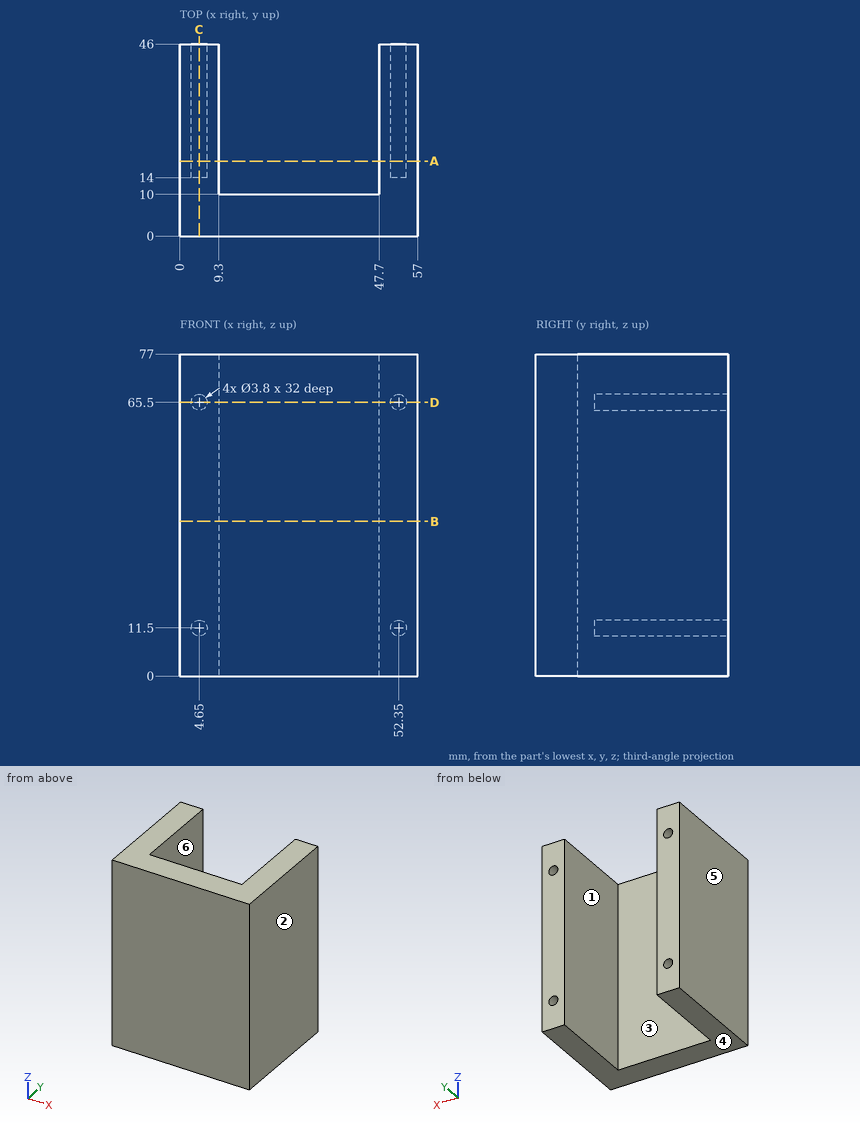
Check sheet for the drawn part. Datum: minimum x, y, z corner. Units: mm. A direction names the side the tool comes from. Give positions to 0.01 mm unless a question says otherwise; leave off trailing zeros. Write each loop counter-clockwise with the first axis right and the second up, starting at its lowest first coordinate (ties: lowest second). Pieces come first, ordered by that corner, then holes.
(1) Access from +Z, -Z, +X, -X, +Y, -Y to the whole of each face (thin tool, end or side, straight path). Record for the marked faces 5 and 6.
(2) Mould release check, pull along X, two halves, no side actions. Record for the marked faces 1, 2, 3 and 4: +X half, -X half, draft (parallel to the pull), parting line (faces both ways), or undercut.
(3) Cross-section at B-B (z = 37). Enter the section's corners in (x, y), plus the area to 3 significant figures.
(4) Cross-section at A-A (y = 18). Enter the section's corners in (x, z), plus the area to 3 significant figures.
(5) Gauge pin test, flat ends, axial feed: pin 1 (4 mm diameter, centred on x = 52, z = 65.5, fed in from +Y); pin 2 (11.5 mm diameter, centred on x = 21.5, z = 49.5, fed in from +Y); pin 3 (2.5 mm diameter, centred on x = 52.35, z = 11.5, fed in from +Y). Record the tip position at first contact, or that the pin passes through.
(6) Cross-section at D-D (z = 65.5). Enter the section's corners in (x, y).
(7) Cross-section at C-C (x = 4.65). Enter the section's corners in (y, z), plus the area to 3 significant figures.
(8) Material ranges on line 1 (X direction, y = 35, z = 65.5); line 2 (X direction, y = 39.5, z = 34.5); line 3 (Z direction, x = 4.5, y = 23.5), recorded low to high.
Worked out:
1. face 5: +Z, -Z, -X, +Y, -Y
1. face 6: +Z, -Z, +Y
2. face 1: undercut
2. face 2: +X half
2. face 3: undercut
2. face 4: draft
3. outline: (0, 0) - (57, 0) - (57, 46) - (47.7, 46) - (47.7, 10) - (9.3, 10) - (9.3, 46) - (0, 46) - close
3. area: 1,240 mm2
4. outline: (0, 0) - (9.3, 0) - (9.3, 77) - (0, 77) - close; (47.7, 0) - (57, 0) - (57, 77) - (47.7, 77) - close; hole circle Ø3.8 at (4.65, 11.5); hole circle Ø3.8 at (4.65, 65.5); hole circle Ø3.8 at (52.35, 11.5); hole circle Ø3.8 at (52.35, 65.5)
4. area: 1,390 mm2
5. pin 1: stops at y = 46
5. pin 2: stops at y = 10
5. pin 3: stops at y = 14
6. outline: (0, 0) - (57, 0) - (57, 46) - (54.25, 46) - (54.25, 14) - (50.45, 14) - (50.45, 46) - (47.7, 46) - (47.7, 10) - (9.3, 10) - (9.3, 46) - (6.55, 46) - (6.55, 14) - (2.75, 14) - (2.75, 46) - (0, 46) - close
7. outline: (0, 0) - (46, 0) - (46, 9.6) - (14, 9.6) - (14, 13.4) - (46, 13.4) - (46, 63.6) - (14, 63.6) - (14, 67.4) - (46, 67.4) - (46, 77) - (0, 77) - close
7. area: 3,300 mm2
8. line 1: x = 0 to 2.75, 6.55 to 9.3, 47.7 to 50.45, 54.25 to 57
8. line 2: x = 0 to 9.3, 47.7 to 57
8. line 3: z = 0 to 9.61, 13.39 to 63.61, 67.39 to 77
